```python
from build123d import *

# Parameters (mm, degrees)
SKETCH2_R           = 17.5
SKETCH2_R_2         = 4.5
SKETCH2_R_3         = 2.2
BOSS_EXTRUDE2_DEPTH = 6
SKETCH3_OUTSIDE_W   = 46.972
SKETCH3_OUTSIDE_H   = 46.972
SKETCH3_OUTSIDE_R   = 15.8
CUT_EXTRUDE1_DEPTH  = 2
CUT_EXTRUDE3_START  = -1.2
CUT_EXTRUDE3_DEPTH  = 1.2


with BuildPart() as part:
    # Sketch2 → Boss-Extrude2 (new body)
    with BuildSketch(Plane(origin=(0, 0, 0), x_dir=(1, 0, 0), z_dir=(0, 1, 0))):
        with Locations(Location((0, 0, 0), (0, 0, 270))):
            Circle(SKETCH2_R)
        with Locations(Location((0, 0, 0), (0, 0, 270))):
            Circle(SKETCH2_R_2, mode=Mode.SUBTRACT)
        with Locations(Location((-8.3, 0, 0), (0, 0, 270))):
            Circle(SKETCH2_R_3, mode=Mode.SUBTRACT)
        with Locations(Location((8.3, 0, 0), (0, 0, 90))):
            Circle(SKETCH2_R_3, mode=Mode.SUBTRACT)
    extrude(amount=BOSS_EXTRUDE2_DEPTH)

    # Sketch3 outside → Cut-Extrude1 (cut)
    with BuildSketch(Plane(origin=(0, 6, 0), x_dir=(1, 0, 0), z_dir=(0, 1, 0))):
        Rectangle(SKETCH3_OUTSIDE_W, SKETCH3_OUTSIDE_H)
        with Locations(Location((0, 0, 0), (0, 0, 270))):
            Circle(SKETCH3_OUTSIDE_R, mode=Mode.SUBTRACT)
    extrude(amount=-CUT_EXTRUDE1_DEPTH, mode=Mode.SUBTRACT)

    # Sketch4 → Cut-Extrude3 (cut)
    with BuildSketch(Plane(origin=(0, 6, 0), x_dir=(1, 0, 0), z_dir=(0, 1, 0)).offset(CUT_EXTRUDE3_START)):
        with BuildLine():
            Line((-9.564911064, -1.8), (-15.697133496, -1.8))
            ThreePointArc((-15.697133496, -1.8), (-15.548872546, -2.805808715), (-15.33623161, -3.8))
            Line((-15.33623161, -3.8), (-2.410394159, -3.8))
            ThreePointArc((-2.410394159, -3.8), (-3.416960076, -2.928204884), (-4.124318125, -1.8))
            Line((-4.124318125, -1.8), (-7.035088936, -1.8))
            ThreePointArc((-7.035088936, -1.8), (-8.3, -2.2), (-9.564911064, -1.8))
        make_face()
        with BuildLine():
            ThreePointArc((15.33623161, -3.8), (15.548872546, -2.805808715), (15.697133496, -1.8))
            Line((15.697133496, -1.8), (9.564911064, -1.8))
            ThreePointArc((9.564911064, -1.8), (8.3, -2.2), (7.035088936, -1.8))
            Line((7.035088936, -1.8), (4.124318125, -1.8))
            ThreePointArc((4.124318125, -1.8), (3.416960076, -2.928204884), (2.410394159, -3.8))
            Line((2.410394159, -3.8), (15.33623161, -3.8))
        make_face()
    extrude(amount=CUT_EXTRUDE3_DEPTH, mode=Mode.SUBTRACT)


solid = part.part
```
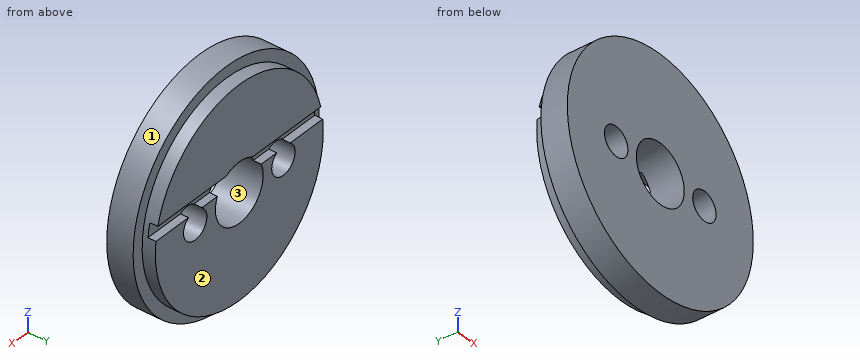
For this review, take the finished solid that the model builds, in its own axes (mm). Face numbers are marked on the shaded views. Round coordinates to 2 decimals unless told otherwise and drop trailing zeros. Write each loop counter-clockwise with the first axis right and the second up, starting at its lowest first coordinate (ties: lowest second). Pieces come first, ordered by that corner, then holes. Notation, with made-up numbers: (0, 46.25) - (11, 46.25) arc R25 ccw to (11, 60.25) - close; hole circle Ø5 at (9, 26.25). An arc over 180 degrees is marked (long way). Use CSV: the item, a comma, the result in double quotes.
1) Add section D-D on y = 3.5. Write out the cut boundary in (x, z).
Conclusion:
outline,"circle Ø35 at (0, 0); hole circle Ø4.4 at (-8.3, 0); hole circle Ø9 at (0, 0); hole circle Ø4.4 at (8.3, 0)"
2) Add section B-B on z = 0. Write out the cut boundary in (x, y).
Conclusion:
outline,"(-17.5, 0) - (-10.5, 0) - (-10.5, 6) - (-15.8, 6) - (-15.8, 4) - (-17.5, 4) - close; (-6.1, 0) - (-4.5, 0) - (-4.5, 6) - (-6.1, 6) - close; (4.5, 0) - (6.1, 0) - (6.1, 6) - (4.5, 6) - close; (10.5, 0) - (17.5, 0) - (17.5, 4) - (15.8, 4) - (15.8, 6) - (10.5, 6) - close"
3) The part is to be moulded in two halves that separate along Z. For the marked faces 1, 2 and 3, say which applies: pulls with the +Z half, pulls with the -Z half, needs draft (parallel to the pull), parting line crosses it, or undercut.
Conclusion:
face 1,"parting line crosses it"
face 2,"needs draft"
face 3,"undercut"
4) Add section C-C on x = -13. Write out the cut boundary in (y, z), and give its area (3 significant figures).
Conclusion:
outline,"(0, -11.72) - (4, -11.72) - (4, -8.98) - (6, -8.98) - (6, 1.8) - (4.8, 1.8) - (4.8, 3.8) - (6, 3.8) - (6, 8.98) - (4, 8.98) - (4, 11.72) - (0, 11.72) - close"
area,"127 mm^2"
5) Wall thickness on line 1 along X through (y, z) = (2, 0); line 2 along X through (y, z) = (4.2, 0); line 3 along Z through (x, y) = (0, 3.15): over which ranges is each line inside the solid? List them lowest first. Write a range as from..to.
Conclusion:
line 1,"x = -17.5..-10.5, -6.1..-4.5, 4.5..6.1, 10.5..17.5"
line 2,"x = -15.8..-10.5, -6.1..-4.5, 4.5..6.1, 10.5..15.8"
line 3,"z = -17.5..-4.5, 4.5..17.5"
6) Clearance check with flat-ended pins moving along their axes: pin 1 Ø0.6 at (x, y) = (-12, 5.5) entering from +Z; pin 2 Ø1.3 at (x, y) = (5, 5) entering from +Z; pin 3 Ø2 at (y, z) = (4.5, 11.5) entering from -X. State where each tip first meets the part, or that it passes through.
Conclusion:
pin 1,"stops at z = 10.62"
pin 2,"stops at z = 15.19"
pin 3,"stops at x = -13.9"
7) Add section A-A on x = 0. Write out the cut boundary in (y, z).
Conclusion:
outline,"(0, -17.5) - (4, -17.5) - (4, -15.8) - (6, -15.8) - (6, -4.5) - (0, -4.5) - close; (0, 4.5) - (6, 4.5) - (6, 15.8) - (4, 15.8) - (4, 17.5) - (0, 17.5) - close"
